Could you check a few things on this model? Use its own coordinates, in mm. Face numbers are marked on the shaded views. A direction names the side the tool comes from. Round coordinates to 2 decimals unless told otherwise and drop trailing zeros. Write each loop counter-clockwise with the first axis right and the second up, starting at its lowest first coordinate (ties: lowest second). Pieces come first, ordered by that corner, then holes.
```python
from build123d import *

# Parameters (mm, degrees)
SKETCH1_W           = 177.8
SKETCH1_H           = 177.8
BOSS_EXTRUDE1_DEPTH = 50.8
SHELL1_T            = -2.54
RIB3_START          = -1.27
RIB3_DEPTH          = 2.54
RIB7_REACH          = 133.37


# Read off the part's stored shape, not the designer's step: Rib3
with BuildPart() as part:
    # Sketch1 → Boss-Extrude1 (new body)
    with BuildSketch(Plane(origin=(0, 0, 0), x_dir=(1, 0, 0), z_dir=(0, 1, 0))):
        Rectangle(SKETCH1_W, SKETCH1_H)
    extrude(amount=BOSS_EXTRUDE1_DEPTH)

    # Shell1
    shell1_openings = [part.faces().sort_by_distance(p)[0] for p in [
        (0, 50.8, 0),
    ]]
    offset(amount=SHELL1_T, openings=shell1_openings, kind=Kind.INTERSECTION)

    # Rib3 outline → Rib3 (add)
    with BuildSketch(Plane.XY.offset(RIB3_START)):
        Polygon((-48.26, 2.54), (-86.36, 40.64), (-86.36, 2.54), align=None)
    rib3 = extrude(amount=RIB3_DEPTH)

    # Mirror1: Rib3 across plane
    add(rib3.mirror(Plane(origin=(0, 0, 0), x_dir=(0, 0, 1), z_dir=(1, 0, 0))))

    # Sketch5 walls → Rib7 (add, up to next)
    with BuildSketch(Plane(origin=(0, 38.1, 0), x_dir=(-1, 0, 0), z_dir=(0, -1, 0)), mode=Mode.PRIVATE) as rib7_sk1:
        with BuildLine():
            Line((-1.905, 218.729821496), (-1.905, 20.868229441))
            ThreePointArc((-1.905, 20.868229441), (-20.955, 0), (-1.905, -20.868229441))
            Line((-1.905, -20.868229441), (-1.905, -218.729821496))
            Line((-1.905, -218.729821496), (1.905, -218.729821496))
            Line((1.905, -218.729821496), (1.905, -17.038837989))
            ThreePointArc((1.905, -17.038837989), (-17.145, 0), (1.905, 17.038837989))
            Line((1.905, 17.038837989), (1.905, 218.729821496))
            Line((1.905, 218.729821496), (-1.905, 218.729821496))
        make_face()
    rib7_tool1 = extrude(rib7_sk1.sketch, amount=RIB7_REACH, mode=Mode.PRIVATE) - part.part
    add(rib7_tool1.solids().sort_by_distance((19.05, 38.1, 0))[0])


solid = part.part
```
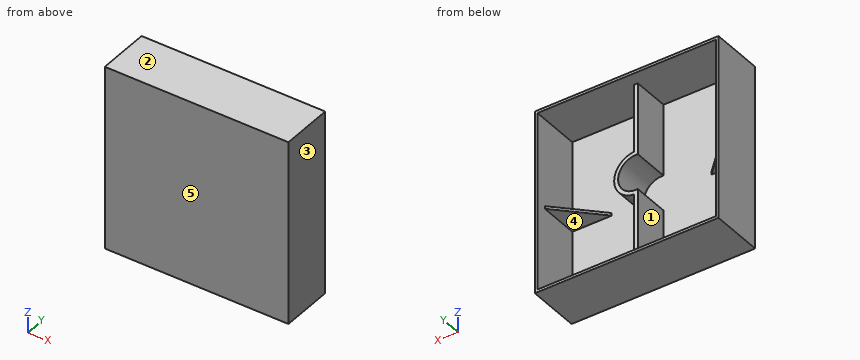
Q1. Imagine slicing it at B-B, the plane x = 52. Write out the boundary of the cut face in (y, z).
Q2. We'd pull the mould along Z, two halves only. Please class the marked faces 1, 2 and 3: pulls with the +Z half, pulls with the -Z half, needs draft (parallel to the pull), parting line crosses it, or undercut.
Q3. Imagine slicing it at C-C, the plane z = -77. Write out the boundary of the cut face in (x, y) (3 decimals).
Q4. Imagine slicing it at D-D, the plane y = 22. Write out the boundary of the cut face in (x, z) (3 decimals), then the cut area to 3 significant figures.
Q5. Imagine slicing it at A-A, the plane y = 7.5. Write out the boundary of the cut face in (x, z) (3 decimals).
Q6. If I drill on L1, parallel to X at y = 28.5, z = -64.5 (3 decimals); L2, parallel to Z at x = -2.5, y = 3, over which ranges is the centre line in solid material (lowest first)?
Q7. On a 3-axis mill with a long thin cutter (end or side, diameter ignored), from which of +Z, -Z, +X, -X, +Y, -Y can I reach the whole of each face in a straight line? I mean the marked faces 4 and 5. Say none if no direction works.
Q8. I'm going to push a flat-ended pin straight in: pin 1 Ø12 at (x, z) = (19, -37) entering from +Y. Where does the tip first touch, or does it pass through?
Results found:
1. outline: (0, -88.9) - (50.8, -88.9) - (50.8, -86.36) - (2.54, -86.36) - (2.54, -1.27) - (6.28, -1.27) - (6.28, 1.27) - (2.54, 1.27) - (2.54, 86.36) - (50.8, 86.36) - (50.8, 88.9) - (0, 88.9) - close
2. face 1: undercut
2. face 2: pulls with the +Z half
2. face 3: needs draft
3. outline: (-88.9, 0) - (88.9, 0) - (88.9, 50.8) - (86.36, 50.8) - (86.36, 2.54) - (1.905, 2.54) - (1.905, 38.1) - (-1.905, 38.1) - (-1.905, 2.54) - (-86.36, 2.54) - (-86.36, 50.8) - (-88.9, 50.8) - close
4. outline: (-88.9, -88.9) - (88.9, -88.9) - (88.9, 88.9) - (-88.9, 88.9) - close; hole (-86.36, -86.36) - (-1.905, -86.36) - (-1.905, -17.039) arc R17.145 ccw (long way) to (-1.905, 17.039) - (-1.905, 86.36) - (-86.36, 86.36) - (-86.36, 1.27) - (-67.72, 1.27) - (-67.72, -1.27) - (-86.36, -1.27) - close; hole (1.905, -86.36) - (86.36, -86.36) - (86.36, -1.27) - (67.72, -1.27) - (67.72, 1.27) - (86.36, 1.27) - (86.36, 86.36) - (1.905, 86.36) - (1.905, 20.868) arc R20.955 cw to (1.905, -20.868) - close
4. area: 2,620 mm2
5. outline: (-88.9, -88.9) - (88.9, -88.9) - (88.9, 88.9) - (-88.9, 88.9) - close; hole (-86.36, -86.36) - (-1.905, -86.36) - (-1.905, -17.039) arc R17.145 ccw (long way) to (-1.905, 17.039) - (-1.905, 86.36) - (-86.36, 86.36) - (-86.36, 1.27) - (-53.22, 1.27) - (-53.22, -1.27) - (-86.36, -1.27) - close; hole (1.905, -86.36) - (86.36, -86.36) - (86.36, -1.27) - (53.22, -1.27) - (53.22, 1.27) - (86.36, 1.27) - (86.36, 86.36) - (1.905, 86.36) - (1.905, 20.868) arc R20.955 cw to (1.905, -20.868) - close
6. L1: x = -88.9 to -86.36, -1.905 to 1.905, 86.36 to 88.9
6. L2: z = -88.9 to -86.36, 86.36 to 88.9
7. face 4: +Y
7. face 5: +Z, -Z, +X, -X, -Y
8. pin 1: stops at y = 2.54
